from build123d import *

# Parameters (mm, degrees)
SKETCH1_R           = 56.769
BOSS_EXTRUDE1_DEPTH = 3.175
SKETCH2_R           = 56.769
SKETCH2_R_2         = 53.594
BOSS_EXTRUDE2_DEPTH = 57.15
SKETCH3_W           = 25.4
SKETCH3_H           = 12.7
CUT_EXTRUDE1_DEPTH  = 101.421832024
CIRPATTERN1_COUNT   = 3
CIRPATTERN1_ANGLE   = 180
SKETCH4_R           = 4.7625
CUT_EXTRUDE2_DEPTH  = 99.547253752


with BuildPart() as part:
    # Sketch1 → Boss-Extrude1 (new body)
    with BuildSketch(Plane(origin=(0, 0, 0), x_dir=(1, 0, 0), z_dir=(0, 1, 0))):
        with Locations(Location((0, 0, 0), (0, 0, 270))):
            Circle(SKETCH1_R)
    extrude(amount=BOSS_EXTRUDE1_DEPTH)

    # Sketch2 → Boss-Extrude2 (add)
    with BuildSketch(Plane(origin=(0, 3.175, 0), x_dir=(1, 0, 0), z_dir=(0, 1, 0))):
        with Locations(Location((0, 0, 0), (0, 0, 270))):
            Circle(SKETCH2_R)
        with Locations(Location((0, 0, 0), (0, 0, 270))):
            Circle(SKETCH2_R_2, mode=Mode.SUBTRACT)
    extrude(amount=BOSS_EXTRUDE2_DEPTH)

    # Sketch3 → Cut-Extrude1 (cut, through all)
    with BuildSketch(Plane(origin=(0, 0, 0), x_dir=(0, 0, -1), z_dir=(1, 0, 0))):
        with Locations((0, 9.525)):
            Rectangle(SKETCH3_W, SKETCH3_H)
    cut_extrude1 = extrude(amount=-CUT_EXTRUDE1_DEPTH, mode=Mode.SUBTRACT)

    # CirPattern1: Cut-Extrude1 ×3 about axis
    cirpattern1_axis = Axis((0, 0, 0), (0, 1, 0))
    for i in range(1, CIRPATTERN1_COUNT):
        add(cut_extrude1.rotate(cirpattern1_axis, i * CIRPATTERN1_ANGLE / (CIRPATTERN1_COUNT - 1)), mode=Mode.SUBTRACT)

    # Sketch4 → Cut-Extrude2 (cut, through all)
    with BuildSketch(Plane(origin=(0, 3.175, 0), x_dir=(1, 0, 0), z_dir=(0, 1, 0))):
        with Locations(Location((0, 45.640625, 0), (0, 0, 270))):
            Circle(SKETCH4_R)
        with Locations(Location((0, 27.384375, 0), (0, 0, 270))):
            Circle(SKETCH4_R)
        with Locations(Location((0, 9.128125, 0), (0, 0, 270))):
            Circle(SKETCH4_R)
        with Locations(Location((0, -9.128125, 0), (0, 0, 270))):
            Circle(SKETCH4_R)
        with Locations(Location((0, -27.384375, 0), (0, 0, 270))):
            Circle(SKETCH4_R)
        with Locations(Location((0, -45.640625, 0), (0, 0, 270))):
            Circle(SKETCH4_R)
    extrude(amount=-CUT_EXTRUDE2_DEPTH, mode=Mode.SUBTRACT)


solid = part.part
Source: CAD feature listing. Evaluate the final solid. Frame: model axes, mm. A direction names the side the tool comes from. Coordinates: 2 decimals unless noted, no trailing zeros. Write each loop counter-clockwise with the first axis right and the second up, starting at its lowest first coordinate (ties: lowest second). Pieces come first, ordered by that corner, then holes. Notation, with made-up numbers: M 16.25,-22 L 38.25,-22 A14 ccw 38.25,-2 Z; hole C 33.5,-3 d2. An arc over 180 degrees is marked long. Use a Markdown table: item, result.
1) First-contact query: pin 1 Ø2 at (x, y) = (-19.5, 14) entering from -Z; pin 2 Ø12 at (x, z) = (41.5, -14.5) entering from +Y (3 decimals); pin 3 Ø3.5 at (y, z) = (6.5, 54) entering from +X. Flat tips, straight axial feed; report the tip coordinate or a pass-through.
Conclusion:
| item | result |
|---|---|
| pin 1 | stops at z = -53.67 |
| pin 2 | stops at y = 3.175 |
| pin 3 | stops at x = 22.2 |
2) Section D-D, the plane z = -37. Output: boundary loops of the cut face in (x, y) (3 decimals).
Conclusion:
| item | result |
|---|---|
| outline | M -43.055,0 L 43.055,0 L 43.055,60.325 L 38.773,60.325 L 38.773,3.175 L -38.773,3.175 L -38.773,60.325 L -43.055,60.325 Z |
3) Reachability of faces 4 (the cylindrical face through (-20.527, 31.35, 49.507)), 5 (the flat face through (12.7, 9, 54)), 6 (the flat face through (54, 9, 12.7)) from +Z, -Z, +X, -X, +Y, -Y: full face, straight path, thin tool, end or side. Return the list, or none.
Conclusion:
| item | result |
|---|---|
| face 4 | +Y |
| face 5 | +Z |
| face 6 | +X, -X |
4) Section A-A, the plane x = 0. Give the number of separate pieces and of enclosed holes in the cut face, then the cut area to 3 significant figures.
Conclusion:
| item | result |
|---|---|
| separate pieces | 8 |
| enclosed holes | 0 |
| area | 502 mm^2 |
5) Mould query, pull axis Z, two halves, no side actions, for faces 1 (the flat face through (-12.7, 9, 54)), 2 (the cylindrical face through (1.431, 1.61, 50.183)), 3 (the cylindrical face through (17.05, 29.74, 54.15)). Classes: pulls with the +Z half, pulls with the -Z half, needs draft (parallel to the pull), parting line crosses it, or undercut.
Conclusion:
| item | result |
|---|---|
| face 1 | needs draft |
| face 2 | undercut |
| face 3 | parting line crosses it |
6) Ray query, L1, parallel to X at y = 24, z = 0; L2, parallel to Y at x = -44.5, z = 6 (3 decimals); L3, parallel to Z at x = 15, y = 57. Return the intervals inside material, ascending.
Conclusion:
| item | result |
|---|---|
| L1 | x = -56.77 to -53.59, 53.59 to 56.77 |
| L2 | y = 0 to 3.175 |
| L3 | z = -54.75 to -51.45, 51.45 to 54.75 |
7) Section C-C, the plane z = 0. Output: boundary loops of the cut face in (x, y) (3 decimals).
Conclusion:
| item | result |
|---|---|
| outline | M -56.769,0 L 56.769,0 L 56.769,3.175 L -56.769,3.175 Z; M -56.769,15.875 L -53.594,15.875 L -53.594,60.325 L -56.769,60.325 Z; M 53.594,15.875 L 56.769,15.875 L 56.769,60.325 L 53.594,60.325 Z |
8) Section B-B, the plane y = 10. Output: boundary loops of the cut face in (x, z), then the cut area to 3 significant figures.
Conclusion:
| item | result |
|---|---|
| outline | M -55.33,-12.7 A56.77 ccw 55.33,-12.7 L 52.07,-12.7 A53.59 cw -52.07,-12.7 Z; M -55.33,12.7 L -52.07,12.7 A53.59 cw -12.7,52.07 L -12.7,55.33 A56.77 ccw Z; M 12.7,52.07 A53.59 cw 52.07,12.7 L 55.33,12.7 A56.77 ccw 12.7,55.33 Z |
| area | 857 mm^2 |
